Geometry: final body of the model. Coordinates: model frame, mm. Face numbers are marked on the shaded views. A direction names the side the tool comes from. Round coordinates to 2 decimals unless told otherwise and drop trailing zeros. Loops run counter-clockwise (first coordinate to the right, second up) from the corner with the lowest first, then second, coordinate; pieces in that order, holes last. Notation, with made-up numbers: (49, -18) - (97, -18) arc R17 ccw to (97, -12) - close; hole circle Ø10 at (-22.5, 71.25). An arc over 180 degrees is marked (long way). Answer as a JSON object with one key per item and string values. Group by question number.
Item 1: Section B-B (z = 40). Return the cut outline in (x, y), plus the area to 3 significant figures.
Item 2: Reachability of the marked faces 4, 5, 6 and 7 from +Z, -Z, +X, -X, +Y, -Y: full face, straight path, thin tool, end or side. Return the list, or none.
Item 3: Section D-D (z = 21.5). Return the cut outline in (x, y), plus the area to 3 significant figures.
Item 4: Line query: line 1 (Y direction, x = 20, z = 2.15); line 2 (Z direction, x = 27, y = 4); line 3 (X direction, y = -13.5, z = 7). Output: solid intervals per line, ascending.
Item 5: Section A-A (x = 20). Return the cut outline in (y, z), plus the area to 3 significant figures.
Item 6: First-contact query: pin 1 (7.5 mm diameter, centred on x = 9.5, z = 14.5, fed in from -Y); pin 2 (8 mm diameter, centred on x = 16, y = -6, fed in from +Z); pin 3 (14 mm diameter, centred on y = 2.5, z = 22.5, fed in from +X); pin 4 (6.5 mm diameter, centred on y = -7.32, z = 40, fed in from -X). Flat tips, straight axial feed; report the tip coordinate or a pass-through.
Item 7: Section C-C (y = 2.5). Return the cut outline in (x, z).
Item 8: Draft query along Z for the marked faces 1, 2 and 3. Return one class per face: released by +Z, released by -Z, zero draft, split by the parting line, or undercut.
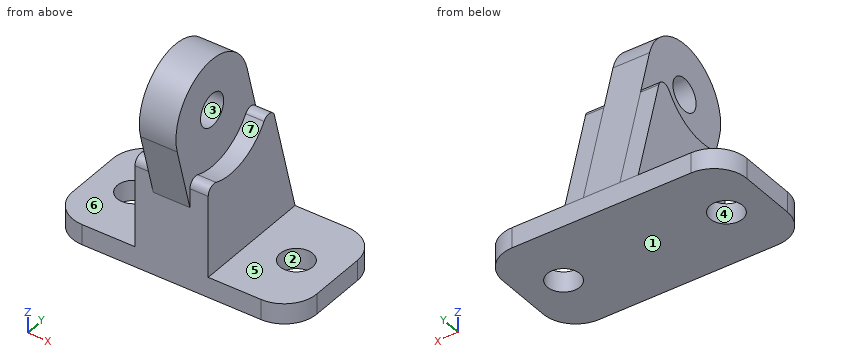
```python
from build123d import *

# Parameters (mm, degrees)
SKETCH2_R                = 4
BOSS_EXTRUDE1_DEPTH      = 5
SKETCH3_R                = 4
BOSS_EXTRUDE2_DEPTH      = 4.5
BOSS_EXTRUDE2_DEPTH_BACK = 4.5
BOSS_EXTRUDE3_DEPTH      = 4.5
BOSS_EXTRUDE3_DEPTH_BACK = 13.5


with BuildPart() as part:
    # Sketch2 → Boss-Extrude1 (new body)
    with BuildSketch(Plane.XY):
        with BuildLine():
            Line((-22, 15), (22, 15))
            ThreePointArc((22, 15), (27.656854249, 12.656854249), (30, 7))
            Line((30, 7), (30, -7))
            ThreePointArc((30, -7), (27.656854249, -12.656854249), (22, -15))
            Line((22, -15), (-22, -15))
            ThreePointArc((-22, -15), (-27.656854249, -12.656854249), (-30, -7))
            Line((-30, -7), (-30, 7))
            ThreePointArc((-30, 7), (-27.656854249, 12.656854249), (-22, 15))
        make_face()
        with Locations((-20, 0)):
            Circle(SKETCH2_R, mode=Mode.SUBTRACT)
        with Locations((20, 0)):
            Circle(SKETCH2_R, mode=Mode.SUBTRACT)
    extrude(amount=BOSS_EXTRUDE1_DEPTH)

    # Sketch3 → Boss-Extrude2 (add, two sides)
    with BuildSketch(Plane(origin=(0, 0, 0), x_dir=(0, 0, -1), z_dir=(1, 0, 0))) as boss_extrude2_sk:
        with BuildLine():
            Line((-36.764761936, -19.393246819), (-5, -10.88190451))
            Line((-5, -10.88190451), (-5, 15))
            Line((-5, 15), (-43.235238064, 4.754898838))
            ThreePointArc((-43.235238064, 4.754898838), (-52.074072829, -10.554412054), (-36.764761936, -19.393246819))
        make_face()
        with Locations((-40, -7.31917399)):
            Circle(SKETCH3_R, mode=Mode.SUBTRACT)
    extrude(amount=BOSS_EXTRUDE2_DEPTH)
    extrude(boss_extrude2_sk.sketch, amount=-BOSS_EXTRUDE2_DEPTH_BACK)

    # Sketch4 → Boss-Extrude3 (add, two sides)
    with BuildSketch(Plane(origin=(4.5, 0, 0), x_dir=(0, 0, -1), z_dir=(1, 0, 0))) as boss_extrude3_sk:
        with BuildLine():
            Line((-25.04245288, -15), (-5, -15))
            Line((-5, -15), (-5, 15))
            Line((-5, 15), (-31.573908753, 7.87954261))
            ThreePointArc((-31.573908753, 7.87954261), (-33.028883618, 6.27753657), (-32.17423683, 4.289332839))
            ThreePointArc((-32.17423683, 4.289332839), (-26.655991742, -3.083912061), (-26.91214627, -12.289896749))
            ThreePointArc((-26.91214627, -12.289896749), (-26.688692003, -14.135736214), (-25.04245288, -15))
        make_face()
    extrude(amount=BOSS_EXTRUDE3_DEPTH)
    extrude(boss_extrude3_sk.sketch, amount=-BOSS_EXTRUDE3_DEPTH_BACK)


solid = part.part
```
Values:
{
 "1": {"outline": "(-4.5, -19.82) - (4.5, -19.82) - (4.5, -11.32) - (-4.5, -11.32) - close; (-4.5, -3.32) - (4.5, -3.32) - (4.5, 5.62) - (-4.5, 5.62) - close", "area": "157 mm^2"},
 "2": {"face 4": "+Z, -Z", "face 5": "+Z, +X, +Y, -Y", "face 6": "+Z, -X, +Y, -Y", "face 7": "+Z, +X"},
 "3": {"outline": "(-9, -15) - (-4.5, -15) - (-4.5, -15.3) - (4.5, -15.3) - (4.5, -15) - (9, -15) - (9, 10.58) - (-9, 10.58) - close", "area": "463 mm^2"},
 "4": {"line 1": "y = -15 to -4, 4 to 15", "line 2": "z = 0 to 5", "line 3": "x = -9 to 9"},
 "5": {"outline": "(-15, 0) - (-4, 0) - (-4, 5) - (-15, 5) - close; (4, 0) - (15, 0) - (15, 5) - (4, 5) - close", "area": "110 mm^2"},
 "6": {"pin 1": "stops at y = -15", "pin 2": "stops at z = 5", "pin 3": "stops at x = 9", "pin 4": "passes through"},
 "7": {"outline": "(-30, 0) - (-23.12, 0) - (-23.12, 5) - (-30, 5) - close; (-16.88, 0) - (16.88, 0) - (16.88, 5) - (9, 5) - (9, 30.02) - (4.5, 30.02) - (4.5, 47.74) - (-4.5, 47.74) - (-4.5, 30.02) - (-9, 30.02) - (-9, 5) - (-16.88, 5) - close; (23.12, 0) - (30, 0) - (30, 5) - (23.12, 5) - close"},
 "8": {"face 1": "released by -Z", "face 2": "zero draft", "face 3": "undercut"}
}
